Verification items for the finished model (mm, model axes). A direction names the side the tool comes from. Coordinates: 2 decimals unless noted, no trailing zeros. Order: outer loops, then holes, each group sorted by start corner. A loop starts at its lowest first (then second) coordinate and runs counter-clockwise, first axis right, second up. Notation, with made-up numbers: M -29.5,-34 L 8.5,-34 A32 ccw 8.5,-7 Z; hole C 39.5,40.5 d11. An arc over 180 degrees is marked long. Return JSON: item names as keys, results as strings. Group by question number.
1. Material ranges on line 1 along Z through (x, y) = (-2.5, -32); line 2 along Y through (x, z) = (-1.25, 5.75); line 3 along X through (y, z) = (-54.5, 5.5), recorded low to high.
2. Section check C-C, the plane y = -16.5. Record the cut outline in (x, z), plus the area to 3 significant figures.
3. Section check A-A, the plane z = 3.75. Record the cut outline in (x, y) (3 decimals), plus the area to 3 significant figures.
4. Section check B-B, the plane y = 1. Record the cut outline in (x, z).
5. Mould release check, pull along Y, two halves, no side actions. Record for faces 1 (the cylindrical face through (7.15, 6.99, 6.93)), 2 (the flat face through (2.5, 11, 9)), 3 (the cylindrical face through (9.268, 9.116, 9.229)): +Y half, -Y half, draft (parallel to the pull), parting line (faces both ways), or undercut.
6. Section check D-D, the plane y = -8. Record the cut outline in (x, z).
7. Gauge pin test, flat ends, axial feed: pin 1 (6 mm diameter, centred on y = -28.5, z = 2.5, fed in from -X); pin 2 (3 mm diameter, centred on x = 8, y = -7, fed in from -Z); pin 3 (1 mm diameter, centred on y = -15, z = 4, fed in from +X); pin 4 (8 mm diameter, centred on x = -10, y = -51, fed in from -Z). Record the tip position at first contact, or that the pin passes through.
8. Set-up check for faces 4 (the flat face through (11, 2.5, 9)), 5 (the cylindrical face through (-0.829, -3.734, 6.821)), 6 (the flat face through (9, -8, 7.75)), 7 (the cylindrical face through (0, 11, 3)): record each of +Z, -Z, +X, -X, +Y, -Y from which the full face is reachable in a straight line by a thin tool's end or side.
```python
from build123d import *

# Parameters (mm, degrees)
CROQUIS1_R                  = 10
SALIENTE_EXTRUIR1_DEPTH     = 3
CROQUIS2_R                  = 11.5
CROQUIS2_R_2                = 10
SALIENTE_EXTRUIR3_DEPTH     = 8
SALIENTE_EXTRUIR4_START     = 3
CROQUIS3_R                  = 11.5
CROQUIS3_R_2                = 10
SALIENTE_EXTRUIR4_DEPTH     = 3
CROQUIS12_W                 = 2.5
CROQUIS12_H                 = 0.622045166
SALIENTE_EXTRUIR6_DEPTH     = 3
CROQUIS13_W                 = 5
CROQUIS13_H                 = 50.27502784
SALIENTE_EXTRUIR7_DEPTH     = 8
CROQUIS15_W                 = 2
CROQUIS15_H                 = 50.27502784
CORTAR_EXTRUIR4_DEPTH       = 8
SALIENTE_EXTRUIR8_DEPTH     = 7
CROQUIS21_R                 = 10
SALIENTE_EXTRUIR9_DEPTH     = 7
CROQUIS22_R                 = 5
CORTAR_EXTRUIR5_DEPTH       = 30
CROQUIS23_R                 = 10
SALIENTE_EXTRUIR10_DEPTH    = 1.25
CORTAR_EXTRUIR6_START       = -1.5
CROQUIS24_R                 = 10
CORTAR_EXTRUIR6_DEPTH       = 1.5
SALIENTE_EXTRUIR11_START    = -3
CROQUIS25_R                 = 13
SALIENTE_EXTRUIR11_DEPTH    = 3
CORTAR_EXTRUIR14_START      = -10
CROQUIS30_R                 = 10
CORTAR_EXTRUIR14_DEPTH      = 10
CROQUIS31_R                 = 11.5
CROQUIS31_R_2               = 10
SALIENTE_EXTRUIR12_DEPTH    = 7.75
CROQUIS32_R                 = 10
SALIENTE_EXTRUIR13_DEPTH    = 10.75
CROQUIS34_R                 = 10
CORTAR_EXTRUIR15_DEPTH      = 7.75
CROQUIS36_R                 = 3.825
SALIENTE_EXTRUIR14_DEPTH    = 7.75
CORTAR_EXTRUIR17_DEPTH      = 77.117731129
CORTAR_EXTRUIR17_DEPTH_BACK = 5.5
SALIENTE_EXTRUIR20_DEPTH    = 9.5
CROQUIS42_W                 = 1.65191017
CROQUIS42_H                 = 5
CORTAR_EXTRUIR18_DEPTH      = 0.25
CORTAR_EXTRUIR19_REACH      = 71.382
CORTAR_EXTRUIR20_REACH      = 71.382
CORTAR_EXTRUIR20_END_RADIUS = 10


with BuildPart() as part:
    # Croquis1 → Saliente-Extruir1 (new body)
    with BuildSketch(Plane.XY):
        Circle(CROQUIS1_R)
    extrude(amount=SALIENTE_EXTRUIR1_DEPTH)



with BuildPart() as body_2:
    # Croquis2 → Saliente-Extruir3 (new body)
    with BuildSketch(Plane.XY.offset(3)):
        Circle(CROQUIS2_R)
        Circle(CROQUIS2_R_2, mode=Mode.SUBTRACT)
    extrude(amount=SALIENTE_EXTRUIR3_DEPTH)


with BuildPart() as part_1:
    add(part.part)

    add(body_2.part)  # Saliente-Extruir4 merges body 2
    # Croquis3 → Saliente-Extruir4 (add)
    with BuildSketch(Plane(origin=(0, 0, 3), x_dir=(-1, 0, 0), z_dir=(0, 0, -1)).offset(SALIENTE_EXTRUIR4_START)):
        with Locations(Location((0, 0, 0), (0, 0, 180))):
            Circle(CROQUIS3_R)
        with Locations(Location((0, 0, 0), (0, 0, 180))):
            Circle(CROQUIS3_R_2, mode=Mode.SUBTRACT)
    extrude(amount=-SALIENTE_EXTRUIR4_DEPTH)

    # Croquis12 → Saliente-Extruir6 (add)
    with BuildSketch(Plane.XY.offset(3)):
        with Locations((-1.25, -11.188977417)):
            Rectangle(CROQUIS12_W, CROQUIS12_H)
        with Locations((1.25, -11.188977417)):
            Rectangle(CROQUIS12_W, CROQUIS12_H)
        Polygon((2.5, -11.5), (2.5, -61.5), (-2.5, -61.5), (-2.5, -11.5), (0, -11.5), align=None)
    extrude(amount=-SALIENTE_EXTRUIR6_DEPTH)

    # Croquis13 → Saliente-Extruir7 (add)
    with BuildSketch(Plane.XY.offset(3)):
        with Locations((0, -36.36248608)):
            Rectangle(CROQUIS13_W, CROQUIS13_H)
    extrude(amount=SALIENTE_EXTRUIR7_DEPTH)

    # Croquis15 → Cortar-Extruir4 (cut)
    with BuildSketch(Plane(origin=(2.5, 0, 0), x_dir=(0, 0, -1), z_dir=(1, 0, 0))):
        with Locations((-10, -36.36248608)):
            Rectangle(CROQUIS15_W, CROQUIS15_H)
        with Locations((-1, -36.36248608)):
            Rectangle(CROQUIS15_W, CROQUIS15_H)
    extrude(amount=-CORTAR_EXTRUIR4_DEPTH, mode=Mode.SUBTRACT)

    # Croquis16 → Saliente-Extruir8 (add)
    with BuildSketch(Plane.XY.offset(9)):
        Polygon((-2.5, -61.5), (-3.5, -61.5), (-3.5, -10.232955502), (3.5, -10.232955502), (3.5, -61.5), (2.5, -61.5), align=None)
    extrude(amount=-SALIENTE_EXTRUIR8_DEPTH)

    # Croquis21 → Saliente-Extruir9 (add)
    with BuildSketch(Plane(origin=(0, 0, 2), x_dir=(-1, 0, 0), z_dir=(0, 0, -1))):
        with Locations((0, -52.72497216)):
            Circle(CROQUIS21_R)
    extrude(amount=-SALIENTE_EXTRUIR9_DEPTH)

    # Croquis22 → Cortar-Extruir5 (cut)
    with BuildSketch(Plane(origin=(0, 0, 2), x_dir=(-1, 0, 0), z_dir=(0, 0, -1))):
        with Locations((0, -52.72497216)):
            Circle(CROQUIS22_R)
    extrude(amount=-CORTAR_EXTRUIR5_DEPTH, mode=Mode.SUBTRACT)

    # Croquis23 → Saliente-Extruir10 (add)
    with BuildSketch(Plane.XY.offset(11)):
        with BuildLine():
            Line((-2.5, -11.22497216), (2.5, -11.22497216))
            ThreePointArc((2.5, -11.22497216), (0, 11.5), (-2.5, -11.22497216))
        make_face()
        Circle(CROQUIS23_R, mode=Mode.SUBTRACT)
    extrude(amount=SALIENTE_EXTRUIR10_DEPTH)

    # Croquis24 → Cortar-Extruir6 (cut)
    with BuildSketch(Plane.XY.offset(12.25).offset(CORTAR_EXTRUIR6_START)):
        with BuildLine():
            Line((-2.5, -11.22497216), (2.5, -11.22497216))
            ThreePointArc((2.5, -11.22497216), (0, 11.5), (-2.5, -11.22497216))
        make_face()
        Circle(CROQUIS24_R, mode=Mode.SUBTRACT)
    extrude(amount=CORTAR_EXTRUIR6_DEPTH, mode=Mode.SUBTRACT)

    # Croquis25 → Saliente-Extruir11 (add)
    with BuildSketch(Plane.XY.offset(10.75).offset(SALIENTE_EXTRUIR11_START)):
        Circle(CROQUIS25_R)
        with BuildLine():
            ThreePointArc((2.5, -11.22497216), (0, 11.5), (-2.5, -11.22497216))
            Line((-2.5, -11.22497216), (2.5, -11.22497216))
        make_face(mode=Mode.SUBTRACT)
    extrude(amount=SALIENTE_EXTRUIR11_DEPTH)

    # Croquis30 → Cortar-Extruir14 (cut)
    with BuildSketch(Plane.XY.offset(3).offset(CORTAR_EXTRUIR14_START)):
        Circle(CROQUIS30_R)
    extrude(amount=CORTAR_EXTRUIR14_DEPTH, mode=Mode.SUBTRACT)

    # Croquis31 → Saliente-Extruir12 (add)
    with BuildSketch(Plane(origin=(0, 0, 0), x_dir=(-1, 0, 0), z_dir=(0, 0, -1))):
        with Locations(Location((0, 0, 0), (0, 0, 180))):
            Circle(CROQUIS31_R)
        with Locations(Location((0, 0, 0), (0, 0, 180))):
            Circle(CROQUIS31_R_2, mode=Mode.SUBTRACT)
    extrude(amount=-SALIENTE_EXTRUIR12_DEPTH)

    # Croquis32 → Saliente-Extruir13 (add)
    with BuildSketch(Plane(origin=(0, 0, 0), x_dir=(-1, 0, 0), z_dir=(0, 0, -1))):
        Circle(CROQUIS32_R)
    extrude(amount=-SALIENTE_EXTRUIR13_DEPTH)

    # Croquis34 → Cortar-Extruir15 (cut)
    with BuildSketch(Plane.XY.offset(10.75)):
        Circle(CROQUIS34_R)
    extrude(amount=-CORTAR_EXTRUIR15_DEPTH, mode=Mode.SUBTRACT)

    # Croquis36 → Saliente-Extruir14 (add)
    with BuildSketch(Plane.XY.offset(3)):
        Circle(CROQUIS36_R)
    extrude(amount=SALIENTE_EXTRUIR14_DEPTH)

    # Croquis40 → Cortar-Extruir17 (cut, two sides: drawn at the far end of the back side and taken through both)
    with BuildSketch(Plane(origin=(0, 11.5, 0), x_dir=(1, 0, 0), z_dir=(0, 1, 0)).offset(-CORTAR_EXTRUIR17_DEPTH_BACK)):
        with BuildLine():
            Line((-2.5, -5.5), (-2.5, -10.75))
            Line((-2.5, -10.75), (0, -10.75))
            Line((0, -10.75), (2.5, -10.75))
            Line((2.5, -10.75), (2.5, -5.5))
            ThreePointArc((2.5, -5.5), (0, -3), (-2.5, -5.5))
        make_face()
        with BuildLine():
            Line((0, -10.75), (-2.5, -10.75))
            ThreePointArc((-2.5, -10.75), (0, -13.25), (2.5, -10.75))
            Line((2.5, -10.75), (0, -10.75))
        make_face()
    extrude(amount=CORTAR_EXTRUIR17_DEPTH + CORTAR_EXTRUIR17_DEPTH_BACK, mode=Mode.SUBTRACT)

    # Croquis7 → Saliente-Extruir20 (add)
    with BuildSketch(Plane.XY.offset(11)):
        Polygon((14.638643631, -2.5), (12.986733461, -2.5), (12.986733461, 0), (12.986733461, 2.5), (14.638643631, 2.5), align=None)
    extrude(amount=-SALIENTE_EXTRUIR20_DEPTH)

    # Croquis42 → Cortar-Extruir18 (cut)
    with BuildSketch(Plane.XY.offset(11)):
        with Locations((13.812688546, 0)):
            Rectangle(CROQUIS42_W, CROQUIS42_H)
    extrude(amount=-CORTAR_EXTRUIR18_DEPTH, mode=Mode.SUBTRACT)

    # Croquis43 → Cortar-Extruir19 (cut, up to next)
    with BuildSketch(Plane(origin=(14.638643631, 0, 0), x_dir=(0, 0, -1), z_dir=(1, 0, 0)), mode=Mode.PRIVATE) as cortar_extruir19_sk1:
        with BuildLine():
            Line((-1.5, 2.5), (-5.5, 2.5))
            ThreePointArc((-5.5, 2.5), (-3, 0), (-5.5, -2.5))
            Line((-5.5, -2.5), (-1.5, -2.5))
            Line((-1.5, -2.5), (-1.5, 2.5))
        make_face()
    cortar_extruir19_tool1 = extrude(cortar_extruir19_sk1.sketch, amount=-CORTAR_EXTRUIR19_REACH, mode=Mode.PRIVATE) & part_1.part
    add(cortar_extruir19_tool1.solids().sort_by_distance((14.638644, 0, 2.594695))[0], mode=Mode.SUBTRACT)

    # Cortar-Extruir20: up to this cylinder (the profile starts outside it)
    cortar_extruir20_end = Plane(origin=(0, 0, 7.121671), z_dir=(0, 0, 1)) * Cylinder(CORTAR_EXTRUIR20_END_RADIUS, 163.764, mode=Mode.PRIVATE)
    # Croquis44 → Cortar-Extruir20 (cut, up to the surface)
    with BuildSketch(Plane(origin=(14.638643631, 0, 0), x_dir=(0, 0, -1), z_dir=(1, 0, 0)), mode=Mode.PRIVATE) as cortar_extruir20_sk1:
        with BuildLine():
            Line((-5.5, 2.5), (-10.75, 2.5))
            Line((-10.75, 2.5), (-10.75, -2.5))
            Line((-10.75, -2.5), (-5.5, -2.5))
            ThreePointArc((-5.5, -2.5), (-3, 0), (-5.5, 2.5))
        make_face()
    cortar_extruir20_tool1 = extrude(cortar_extruir20_sk1.sketch, amount=-CORTAR_EXTRUIR20_REACH, mode=Mode.PRIVATE) - cortar_extruir20_end
    add(cortar_extruir20_tool1.solids().sort_by_distance((14.638644, 0, 7.121671))[0], mode=Mode.SUBTRACT)


solid = part_1.part
```
Answers follow:
{
 "1": {"line 1": "2 to 9", "line 2": "-62.65 to -57.57, -47.88 to -9.92, -3.61 to 3.61", "line 3": "-9.84 to -4.67, 4.67 to 9.84"},
 "2": {"outline": "M -3.5,2 L 3.5,2 L 3.5,9 L -3.5,9 Z", "area": "49.0 mm^2"},
 "3": {"outline": "C 0,0 d7.65; M -3.5,-43.357 A10 ccw long 3.5,-43.357 L 3.5,-10.954 A11.5 ccw 11.361,-1.785 L 9.839,-1.785 A10 cw long -1.785,9.839 L -1.785,11.361 A11.5 ccw -3.5,-10.954 Z; M 1.785,9.839 A10 cw 9.839,1.785 L 11.361,1.785 A11.5 ccw 1.785,11.361 Z; hole C 0,-52.725 d10", "area": "593 mm^2"},
 "4": {"outline": "M -12.96,7.75 L -11.46,7.75 L -11.46,0 L 11.46,0 L 11.46,3.21 L 9.95,3.21 L 9.95,3 L 3.69,3 L 3.69,10.75 L -3.69,10.75 L -3.69,3 L -9.95,3 L -9.95,10.75 L -12.96,10.75 Z"},
 "5": {"face 1": "undercut", "face 2": "draft", "face 3": "+Y half"},
 "6": {"outline": "M -10.25,7.75 L -8.26,7.75 L -8.26,0 L 8.26,0 L 8.26,7.75 L 10.25,7.75 L 10.25,10.75 L 6,10.75 L 6,3 L -6,3 L -6,10.75 L -10.25,10.75 Z"},
 "7": {"pin 1": "x = -3.5", "pin 2": "z = 0", "pin 3": "x = 3.5", "pin 4": "z = 2"},
 "8": {"face 4": "+Z, +X", "face 5": "+Z", "face 6": "-Z, +X", "face 7": "+Z, +Y"}
}
